Check sheet for the modelled part. Datum: model origin and axes. Units: mm. Coordinates: 2 decimals unless noted, no trailing zeros. Loops run counter-clockwise (first coordinate to the right, second up) from the corner with the lowest first, then second, coordinate; pieces in that order, holes last. Notation, with made-up numbers: M 12.25,69 L 17.25,69 A15 cw 17.25,80 Z; hole C 23.5,-20.5 d9. An arc over 180 degrees is marked long. Answer in a Markdown table with one row per item. Add a question column.
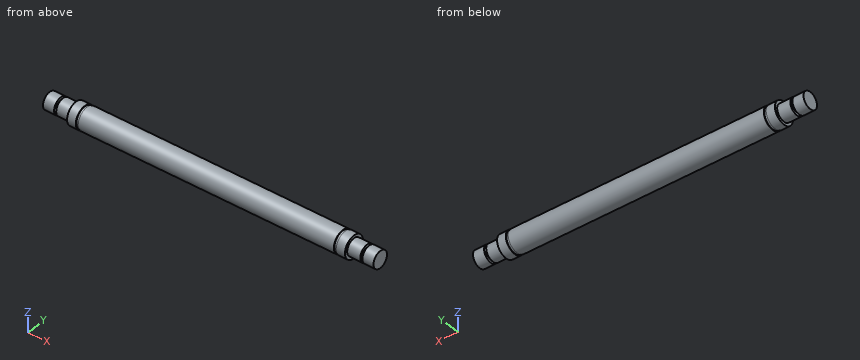
Autodesk Fusion 360 part; units mm, degrees
sketch "Sketch1" plane through (0, 0, 0) normal (1, 0, 0) x (0, 1, 0)
  circle A0 centre (0, 0) radius 3
  dimension "d1" = 6
extrude "Extrude1" add sketch "Sketch1" along normal blind 8
sketch "Sketch2" plane through (8, 0, 0) normal (1, 0, 0) x (0, 1, 0)
  circle A0 centre (0, 0) radius 3
  circle A1 centre (0, 0) radius 4
  dimension "d4" = 8
extrude "Extrude2" add sketch "Sketch2" along normal blind 3.15 contours A0 | A1
sketch "Sketch3" plane through (11.15, 0, 0) normal (1, 0, 0) x (0, 1, 0)
  circle A0 centre (0, 0) radius 4
  circle A1 centre (0, 0) radius 3.775
  dimension "d7" = 7.55
extrude "Extrude3" add sketch "Sketch3" along normal blind 0.85 contours A1
sketch "Sketch4" plane through (12, 0, 0) normal (1, 0, 0) x (0, 1, 0)
  circle A0 centre (0, 0) radius 3.775
  circle A1 centre (0, 0) radius 4
  dimension "d10" = 8
extrude "Extrude4" add sketch "Sketch4" along normal blind 92 contours A0 | A1
sketch "Sketch5" plane through (104, 0, 0) normal (1, 0, 0) x (0, 1, 0)
  circle A0 centre (0, 0) radius 4
  circle A1 centre (0, 0) radius 3.775
  dimension "d13" = 7.55
extrude "Extrude5" add sketch "Sketch5" along normal blind 0.85 contours A1
sketch "Sketch6" plane through (104.85, 0, 0) normal (1, 0, 0) x (0, 1, 0)
  circle A0 centre (0, 0) radius 3.775
  circle A1 centre (0, 0) radius 4
  dimension "d16" = 8
extrude "Extrude6" add sketch "Sketch6" along normal blind 3.15 contours A0 | A1
extrude "Extrude8" cut 1 faces at (0, -1.1591, 0.5829) along direction (1, 0, 0) blind 8
sketch "Sketch8" plane through (8, 0, 0) normal (-1, 0, 0) x (0, -1, 0)
  circle A0 centre (0, 0) radius 4
  circle A1 centre (0, 0) radius 3
  dimension "d24" = 6
extrude "Extrude9" add sketch "Sketch8" along normal blind 4.72 contours A1
sketch "Sketch9" plane through (3.28, 0, 0) normal (-1, 0, 0) x (0, -1, 0)
  circle A0 centre (0, 0) radius 3
  circle A1 centre (0, 0) radius 2
  dimension "d27" = 4
extrude "Extrude10" add sketch "Sketch9" along normal blind 0.75 contours A1
sketch "Sketch10" plane through (2.53, 0, 0) normal (-1, 0, 0) x (0, -1, 0)
  circle A0 centre (0, 0) radius 2
  circle A1 centre (0, 0) radius 3
  dimension "d30" = 6
extrude "Extrude11" add sketch "Sketch10" along normal blind 4 contours A0 | A1
sketch "Sketch11" plane through (108, 0, 0) normal (1, 0, 0) x (0, 1, 0)
  circle A0 centre (0, 0) radius 4
  circle A1 centre (0, 0) radius 3
  dimension "d33" = 6
extrude "Extrude12" add sketch "Sketch11" along normal blind 4.72 contours A1
sketch "Sketch12" plane through (112.72, 0, 0) normal (1, 0, 0) x (0, 1, 0)
  circle A0 centre (0, 0) radius 3
  circle A1 centre (0, 0) radius 2
  dimension "d36" = 4
extrude "Extrude13" add sketch "Sketch12" along normal blind 0.75 contours A1
sketch "Sketch13" plane through (113.47, 0, 0) normal (1, 0, 0) x (0, 1, 0)
  circle A0 centre (0, 0) radius 2
  circle A1 centre (0, 0) radius 3
  dimension "d39" = 6
extrude "Extrude14" add sketch "Sketch13" along normal blind 4 contours A0 | A1
equation "d17 = 100 mm - 96.85 mm"
Q1. Go/stop test with flat-tipped pins: pin 1 (1 mm diameter, centred on y = 3, z = -3, fed in from -X); pin 2 (1 mm diameter, centred on x = 68, z = -1.5, fed in from +Y); pin 3 (2 mm diameter, centred on x = 55.5, z = 2, fed in from -Y). Record where each tip stops, or that it passes through.
Q2. Cross-section at A-A (x = 61). Record the cut outline in (y, z), plus the area to 3 significant figures.
Q3. Thickness scan on L1, parallel to X at y = 1.75, z = -2; L2, parallel to Z at x = 74, y = -0.25; L3, parallel to X at y = -2.5, z = 2.5. Record the ranges inside material, lowest first.
Answer key:
| question | item | result |
|---|---|---|
| 1 | pin 1 | x = 8 |
| 1 | pin 2 | y = 3.87 |
| 1 | pin 3 | y = -3.87 |
| 2 | outline | C 0,0 d8 |
| 2 | area | 50.3 mm^2 |
| 3 | L1 | -1.47 to 2.53, 3.28 to 112.72, 113.47 to 117.47 |
| 3 | L2 | -3.99 to 3.99 |
| 3 | L3 | 8 to 108 |
